Input: part model. Units: mm. Frame: model coordinates. A direction names the side the tool comes from. Round coordinates to 2 decimals unless told otherwise and drop trailing zeros. Loops run counter-clockwise (first coordinate to the right, second up) from the corner with the lowest first, then second, coordinate; pieces in that order, holes last.
1) First-contact query: pin 1 (6 mm diameter, centred on x = -4, z = 32.5, fed in from -Y); pin 2 (6 mm diameter, centred on x = 3.5, z = 31, fed in from -Y); pin 3 (2.5 mm diameter, centred on x = 2, y = -12.5, fed in from +Z). Flat tips, straight axial feed; report the tip coordinate or a pass-through.
2) Section C-C, the plane x = 2.25. Return loops of the section in (y, z).
3) Section D-D, the plane z = 33.5. Return loops of the section in (x, y).
4) Draft query along Y for faces 4 (the face through (-0.275, -19.562, 23.716)), 5 (the face through (4, 0, 34)), 6 (the face through (-6.261, -2.697, 32.775)). Return one class per face: pulls with the +Y half, pulls with the -Y half, needs draft (parallel to the pull), parting line crosses it, or undercut.
5) Ray query, line 1 along Y through (x, z) = (1, 26.5) (3 decimals); line 2 along X through (y, z) = (-3, 32.75); line 3 along Y through (x, z) = (3.75, 29.25). Return the intervals inside material, ascending.
6) Section A-A, the plane z = 23.75. Return loops of the section in (x, y) (3 decimals).
7) Access query for faces 1 (the face through (4, -13, 26.534)), 2 (the face through (3.75, -17.72, 23.72)), 3 (the face through (7.62, -7, 28)). Directions: +Z, -Z, +X, -X, +Y, -Y. A direction counts if a zero-diameter tool reaches every point of the face in a straight line with its end or side. Return the directions, or none.
8) Section B-B, the plane y = -16.75. Return loops of the section in (x, z), and give its area (3 significant figures).
from build123d import *

# Parameters (mm, degrees)
F0_W      = 5.08
F0_H      = 12.7
F1_DEPTH  = 5.08
F2_W      = 5.08
F2_H      = 3.81
F3_DEPTH  = 6.35
F4_R      = 5.08
F5_R      = 2.7121475218
F6_DEPTH  = 3.81
F7_R      = 1.9253373718
F8_DEPTH  = 3.81
F9_W      = 5.3527112813
F9_H      = 1.6279429131
F10_DEPTH = 3.81
F11_SCALE = 1.5
F12_R     = 2.413
F13_DEPTH = 20.32


with BuildPart() as f1:
    # F0 (on Front) → F1 (new body)
    with BuildSketch(Plane.XZ):
        with Locations((2.54, 20.2292869008)):
            Rectangle(F0_W, F0_H)
    extrude(amount=F1_DEPTH)

    # F2 (on face) → F3 (join)
    with BuildSketch(Plane.XZ.offset(5.08)):
        with Locations((2.54, 15.7842869008)):
            Rectangle(F2_W, F2_H)
    extrude(amount=F3_DEPTH)

    # F4
    f4_edges = [f1.edges().sort_by_distance(p)[0] for p in [
        (2.54, 0, 13.879287),
    ]]
    fillet(f4_edges, radius=F4_R)

    # F5 (on face) → F6 (join)
    with BuildSketch(Plane.XY.offset(17.6892869008)):
        with Locations((2.4383503072, -13.7368525874)):
            Circle(F5_R)
    extrude(amount=-F6_DEPTH)

    # F7 (on face) → F8 (cut)
    with BuildSketch(Plane.XY.offset(17.6892869008)):
        with Locations((2.4383503072, -13.7368525874)):
            Circle(F7_R)
    extrude(amount=-F8_DEPTH, mode=Mode.SUBTRACT)

    # F9 (on face) → F10 (cut)
    with BuildSketch(Plane.XY.offset(17.6892869008)):
        with Locations((2.7606785416, -15.8977832678)):
            Rectangle(F9_W, F9_H)
    extrude(amount=-F10_DEPTH, mode=Mode.SUBTRACT)


with BuildPart() as f1_1:
    # F11: moved
    add(f1.part.scale(F11_SCALE))

    # F12 (on face) → F13 (join)
    with BuildSketch(Plane.YZ.offset(7.62)):
        with Locations((-3.81, 34.9159303513)):
            Circle(F12_R)
    extrude(amount=-F13_DEPTH)


solid = f1_1.part
Final values:
1. pin 1: stops at y = -6.22
1. pin 2: stops at y = -7.62
1. pin 3: stops at z = 26.53
2. outline: (-18.08, 20.82) - (-7.62, 20.82) arc R7.62 ccw to (0, 28.44) - (0, 39.87) - (-7.62, 39.87) - (-7.62, 26.53) - (-18.08, 26.53) - close
3. outline: (-12.7, -5.76) - (0, -5.76) - (0, -7.62) - (7.62, -7.62) - (7.62, 0) - (0, 0) - (0, -1.86) - (-12.7, -1.86) - close
4. face 4: undercut
4. face 5: pulls with the +Y half
4. face 6: parting line crosses it
5. line 1: y = -22.626 to -21.736, -19.475 to -17.525, -17.145 to -0.251
5. line 2: x = -12.7 to 7.62
5. line 3: y = -7.62 to 0
6. outline: (0, -17.145) - (1.518, -17.145) arc R4.068 ccw to (0.126, -22.626) - (1.594, -22.626) arc R2.888 cw (long way) to (5.721, -22.626) - (7.189, -22.626) arc R4.068 ccw to (5.797, -17.145) - (7.62, -17.145) - (7.62, -1.613) - (0, -1.613) - close
7. face 1: +Z, +X, -X, -Y
7. face 2: +Z, -Z
7. face 3: +Z, -Z, +X, +Y
8. outline: (0, 20.82) - (7.62, 20.82) - (7.62, 26.53) - (0, 26.53) - close
8. area: 43.5 mm2
